Could you check a few things on this drawing? It's one solid part, dimensions in mm from its lowest x, y, z. A direction names the side the tool comes from. Give positions to 0.01 mm unless a question says otherwise; leave off trailing zeros. Order: outer loops, then holes, each group sorted by start corner. A loop starts at its lowest first (then second) coordinate and runs counter-clockwise, first axis right, second up.
(1) On a 3-axis mill with a long thin cutter (end or side, diameter ignored), from which of +Z, -Z, +X, -X, +Y, -Y can I reach the whole of each face in a straight line? I mean the marked faces 1, 2 and 3. Say none if no direction works.
(2) Imagine slicing it at D-D, the plane z = 64. Write out the boundary of the cut face in (x, y), then the cut area to 3 significant figures.
(3) Imagine slicing it at C-C, the plane z = 18.5. Write out the boundary of the cut face in (x, y).
(4) If we mould it in two halves opening along X, with no side actions, what happens to the marked faces 4, 5, 6 and 7? For each: released by +X, released by -X, zero draft, split by the parting line, or undercut.
(5) Will these pins go through, and if not, where does the flat tip stop? pin 1 (4 mm diameter, centred on y = 29.5, z = 60, fed in from +X); pin 2 (3 mm diameter, centred on x = 36.5, z = 24, fed in from +Y); pin 3 (2 mm diameter, centred on x = 85.5, y = 52, fed in from +Z).
(6) If I drill on probe 1 along Y at (x, z) = (60, 12); probe 2 along Y at (x, z) = (60, 20.5); probe 3 along Y at (x, z) = (62, 45), over which ranges is the centre line in solid material (lowest first)?
(7) Imagine slicing it at A-A, the plane x = 60. Write out the boundary of the cut face in (y, z), then the cut area to 3 significant figures.
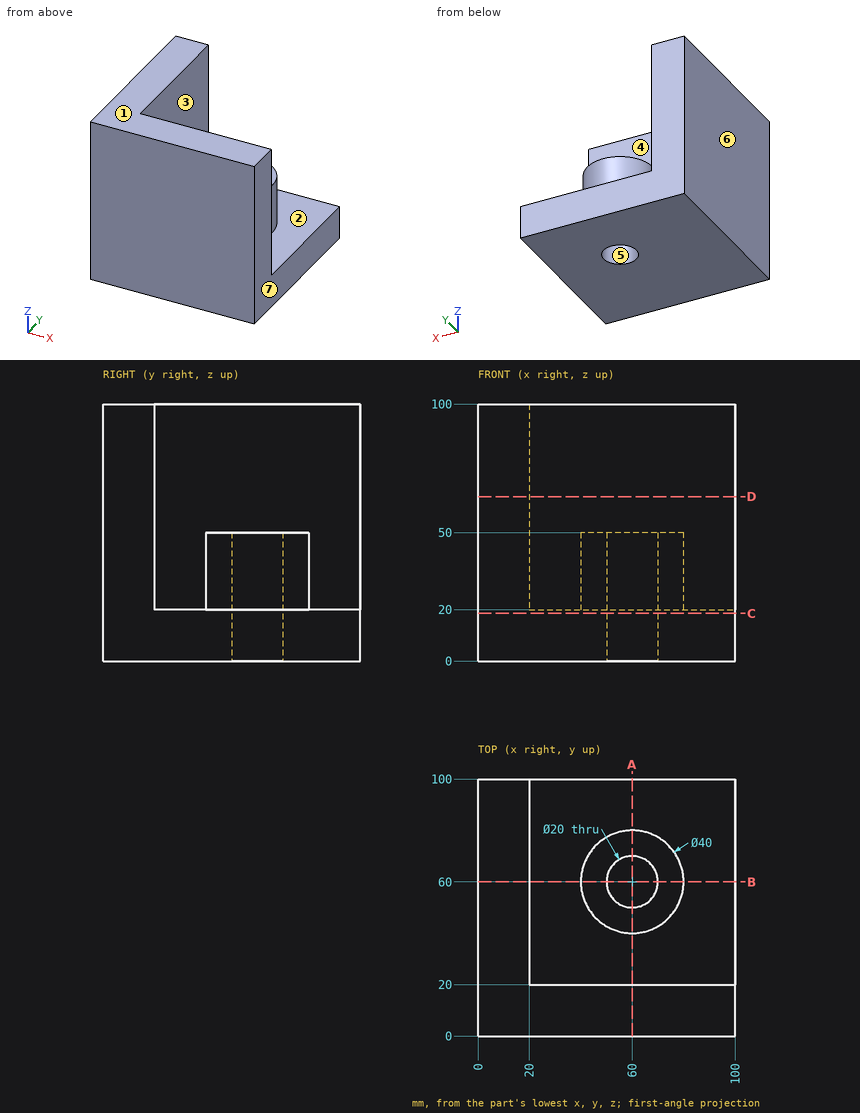
Answer block:
1. face 1: +Z, +X, -X, +Y, -Y
1. face 2: +Z
1. face 3: +Z, +Y
2. outline: (0, 0) - (100, 0) - (100, 20) - (20, 20) - (20, 100) - (0, 100) - close
2. area: 3,600 mm2
3. outline: (0, 0) - (100, 0) - (100, 100) - (0, 100) - close; hole circle Ø20 at (60, 60)
4. face 4: zero draft
4. face 5: undercut
4. face 6: released by -X
4. face 7: released by +X
5. pin 1: stops at x = 20
5. pin 2: stops at y = 20
5. pin 3: stops at z = 20
6. probe 1: y = 0 to 50, 70 to 100
6. probe 2: y = 0 to 20, 40 to 50, 70 to 80
6. probe 3: y = 0 to 20, 40.1 to 50.2, 69.8 to 79.9
7. outline: (0, 0) - (50, 0) - (50, 50) - (40, 50) - (40, 20) - (20, 20) - (20, 100) - (0, 100) - close; (70, 0) - (100, 0) - (100, 20) - (80, 20) - (80, 50) - (70, 50) - close
7. area: 3,800 mm2
